Autodesk Inventor part; units mm, degrees
ref_plane "YZ Plane" through (0, 0, 0) normal (1, 0, 0) x (0, 1, 0)
ref_plane "XZ Plane" through (0, 0, 0) normal (0, 1, 0) x (-1, 0, 0)
ref_plane "XY Plane" through (0, 0, 0) normal (0, 0, 1) x (1, 0, 0)
sketch "Boceto1" plane through (0, 0, 0) normal (0, 1, 0) x (-1, 0, 0)
  line L0 (0, 0) -> (-50, 0)
  line L1 (-50, 0) -> (-50, -50)
  line L2 (-50, -50) -> (0, -50)
  line L3 (0, -50) -> (0, 0)
  dimension "d0" = 50
  dimension "d1" = 50
extrude "Extrusión1" add sketch "Boceto1" along normal blind 5
sketch "Boceto2" plane through (0, 5, 0) normal (0, 1, 0) x (1, 0, 0)
  circle A0 centre (10, 10) radius 2.5
  line L0 (0, 50) -> (0, 0)
  line L1 (0, 0) -> (50, 0)
  circle A1 centre (10, 40) radius 2.5
  circle A2 centre (40, 10) radius 2.5
  circle A3 centre (40, 40) radius 2.5
  line L2 (50, 50) -> (0, 50)
  line L3 (50, 0) -> (50, 50)
  dimension "d4" = 5
  dimension "d5" = 10
  dimension "d6" = 10
  dimension "d7" = 5
  dimension "d8" = 5
  dimension "d9" = 5
  dimension "d10" = 10
  dimension "d11" = 10
  dimension "d12" = 10
  dimension "d13" = 10
  dimension "d14" = 10
  dimension "d15" = 10
extrude "Extrusión2" add sketch "Boceto2" along normal blind 75 contours A0 | A1 | A2 | A3
sketch "Boceto3" plane through (10, 80, -10) normal (0, 1, 0) x (1, 0, 0)
  line L0 (-10, -10) -> (40, -10)
  line L1 (40, 40) -> (-10, 40)
  line L2 (-10, -10) -> (40, -10)
  line L3 (40, -10) -> (40, 40)
  line L4 (40, 40) -> (-10, 40)
  line L5 (-10, 40) -> (-10, -10)
extrude "Extrusión3" add sketch "Boceto3" along normal blind 5
sketch "Boceto4" plane through (10, 85, -10) normal (0, 1, 0) x (1, 0, 0)
  circle A0 centre (15, 15) radius 2.5
  line L0 (40, 40) -> (-10, 40)
  line L1 (-10, 40) -> (-10, -10)
  dimension "d20" = 5
  dimension "d21" = 25
  dimension "d22" = 25
extrude "Extrusión4" cut sketch "Boceto4" against normal blind 5
thread "Rosca1"
sketch "Boceto7" plane through (50, 80, -50) normal (0, 0, -1) x (-1, 0, 0)
  line L0 (0, 5) -> (50, 5)
  line L1 (25, 5) -> (75, 5)
  line L2 (75, 5) -> (75, 0)
  line L3 (75, 0) -> (25, 0)
  line L4 (25, 0) -> (25, 5)
  point P0 (50, -80)
  dimension "d34" = 50
  dimension "d35" = 5
extrude "Extrusión7" add sketch "Boceto7" along normal blind 200
sketch "Boceto8" plane through (0, 80, 0) normal (-1, 0, 0) x (0, 0, 1)
  line L0 (-50, 5) -> (0, 5)
  line L1 (-50, 0) -> (-250, 0)
  line L2 (-25, 5) -> (-75, 5)
  line L3 (-75, 5) -> (-75, 0)
  line L4 (-75, 0) -> (-25, 0)
  line L5 (-25, 0) -> (-25, 5)
  point P0 (0, -80)
  dimension "d38" = 50
extrude "Extrusión8" add sketch "Boceto8" along normal blind 200
sketch "Boceto9" plane through (10, 85, -10) normal (0, 1, 0) x (1, 0, 0)
  circle A0 centre (15, 30) radius 2.5
  circle A1 centre (15, 15) radius 2.5
  point P0 (-10, -10)
  dimension "d41" = 5
  dimension "d42" = 15
  dimension "d43" = 0
extrude "Extrusión9" cut sketch "Boceto9" against normal blind 10 contours A0
thread "Rosca2"
sketch "Boceto10" plane through (10, 80, -10) normal (0, -1, 0) x (1, 0, 0)
  circle A0 centre (5, -230) radius 2.5
  circle A1 centre (-25, -230) radius 2.5
  circle A2 centre (-25, -200) radius 2.5
  circle A3 centre (5, -200) radius 2.5
  line L0 (15, -240) -> (-35, -240)
  line L1 (15, -40) -> (15, -240)
  line L2 (-35, -65) -> (-35, -240)
  line L3 (15, -40) -> (15, -240) construction
  line L4 (15, -190) -> (-35, -190) construction
  point P0 (-10, 10)
  dimension "d48" = 5
  dimension "d49" = 5
  dimension "d50" = 5
  dimension "d51" = 5
  dimension "d52" = 10
  dimension "d53" = 10
  dimension "d54" = 10
  dimension "d55" = 10
  dimension "d56" = 50
  dimension "d57" = 10
  dimension "d58" = 10
  dimension "d59" = 10
  dimension "d60" = 10
extrude "Extrusión10" add sketch "Boceto10" along normal blind 75
sketch "Boceto11" plane through (-15, 5, -240) normal (0, -1, 0) x (1, 0, 0)
  circle A0 centre (-145, 175) radius 2.5
  circle A1 centre (-175, 175) radius 2.5
  circle A2 centre (-145, 205) radius 2.5
  circle A3 centre (-175, 205) radius 2.5
  line L0 (15, 215) -> (-185, 215)
  line L1 (-185, 165) -> (-185, 215)
  line L2 (-10, 165) -> (-185, 165) construction
  line L3 (-135, 165) -> (-135, 215) construction
  point P0 (15, 240)
  dimension "d63" = 5
  dimension "d64" = 5
  dimension "d65" = 5
  dimension "d66" = 5
  dimension "d67" = 10
  dimension "d68" = 10
  dimension "d69" = 50
  dimension "d70" = 10
  dimension "d71" = 10
  dimension "d72" = 10
  dimension "d73" = 10
  dimension "d74" = 10
  dimension "d75" = 10
extrude "Extrusión11" add sketch "Boceto11" against normal blind 75
sketch "Boceto12" plane through (-190, 5, -35) normal (0, -1, 0) x (1, 0, 0)
  line L0 (215, -15) -> (215, -215)
  line L1 (165, -40) -> (165, -215)
  line L2 (215, -215) -> (165, -215)
  line L3 (165, -215) -> (165, -165)
  line L4 (165, -165) -> (215, -165)
  line L5 (215, -165) -> (215, -215)
  line L6 (165, -40) -> (-10, -40)
  line L7 (190, 10) -> (-10, 10)
  line L8 (-10, -40) -> (40, -40)
  line L9 (40, -40) -> (40, 10)
  line L10 (40, 10) -> (-10, 10)
  line L11 (-10, 10) -> (-10, -40)
  point P0 (190, 35)
  dimension "d78" = 50
  dimension "d79" = 50
extrude "Extrusión12" add sketch "Boceto12" along normal blind 5
properties part number "Soporte - C15_3DPrint"
The model under review builds one solid part; all positions refer to its coordinate system, in mm. A direction names the side the tool comes from. Round coordinates to 2 decimals unless told otherwise and drop trailing zeros. Loops run counter-clockwise (first coordinate to the right, second up) from the corner with the lowest first, then second, coordinate; pieces in that order, holes last. Notation, with made-up numbers: M 4.25,3 L 52.25,3 A18 cw 52.25,24 Z; hole C -3.5,40 d3. An arc over 180 degrees is marked long. Answer as CSV lines item,"result".
1. We need section A-A (y = 35). Count the separate pieces of the cut face and the enclosed holes in it, plus the area to 3 significant figures.
Outcome:
separate pieces,"12"
enclosed holes,"0"
area,"236 mm2"
2. We need section B-B (x = -52). Give the boundary of the cut face in (y, z), plus the area to 3 significant figures.
Outcome:
outline,"M 80,-75 L 85,-75 L 85,-25 L 80,-25 Z"
area,"250 mm2"
3. Draft analysis for pull direction Y (two halves, no side actions). For faces 3 (the face through (0, 5, -225)), 4 (the face through (-175, 0, -50)), 5 (the face through (-45, 85, -71)), 6 (the face through (-45, 80, -71)), state which applies: pulls with the +Y half, pulls with the -Y half, needs draft (parallel to the pull), parting line crosses it, or undercut.
Outcome:
face 3,"undercut"
face 4,"pulls with the -Y half"
face 5,"pulls with the +Y half"
face 6,"undercut"
4. Insertion check: pin 1 Ø5.5 at (x, y) = (10, 1.5) entering from +Z; pin 2 Ø2.5 at (y, z) = (83.5, -12.5) entering from -X; pin 3 Ø1.5 at (y, z) = (3.5, -236) entering from +X; pin 4 Ø1.5 at (x, y) = (34.5, 2.5) entering from -Z. Each pin has a flat end and moves straight along its axis. Give the tip position at first contact, or say it passes through.
Outcome:
pin 1,"stops at z = 0"
pin 2,"stops at x = 0"
pin 3,"stops at x = 25"
pin 4,"stops at z = -50"
5. We need section C-C (z = -146.5). Give the boundary of the cut face in (x, y), plus the area to 3 significant figures.
Outcome:
outline,"M -25,80 L 25,80 L 25,85 L -25,85 Z"
area,"250 mm2"
6. To check wall thickness, follow L1, parallel to X at y = 81, z = -40; L2, parallel to Y at x = -21, z = -109; L3, parallel to X at y = 44, z = -12. State the ranges of each line that lie inside material, in increasing order. Write a range as [from, to].
Outcome:
L1,"x = [-200, 22.5], [27.5, 50]"
L2,"y = [80, 85]"
L3,"x = [8.5, 11.5], [38.5, 41.5]"
7. For faces 1 (the face through (25, 0, -25)), 2 (the face through (-175, 5, -50)), list the 3-axis set-ups (+Z, -Z, +X, -X, +Y, -Y) from which the entire face can be reached by the end or side of a thin tool; tool diameter is ignored.
Outcome:
face 1,"+Z, -Z, +X, -X, -Y"
face 2,"none"
